```python
from build123d import *

# Parameters (mm, degrees)
SKETCH1_R             = 1.1
SKETCH1_R_2           = 3.75
BOSS_EXTRUDE1_DEPTH   = 2
F_1_0MM_DOWEL_HOLE1_D = 1
FILLET1_R             = 1


with BuildPart() as part:
    # Sketch1 → Boss-Extrude1 (new body)
    with BuildSketch(Plane.XY):
        with BuildLine():
            Line((-19.5, 2.7), (-6.306155873, 4.504985917))
            ThreePointArc((-6.306155873, 4.504985917), (0, 7.75), (6.306155873, 4.504985917))
            Line((6.306155873, 4.504985917), (19.5, 2.7))
            ThreePointArc((19.5, 2.7), (22.2, 0), (19.5, -2.7))
            Line((19.5, -2.7), (6.306155873, -4.504985917))
            ThreePointArc((6.306155873, -4.504985917), (0, -7.75), (-6.306155873, -4.504985917))
            Line((-6.306155873, -4.504985917), (-19.5, -2.7))
            ThreePointArc((-19.5, -2.7), (-22.2, 0), (-19.5, 2.7))
        make_face()
        with Locations((-19.5, 0)):
            Circle(SKETCH1_R, mode=Mode.SUBTRACT)
        with Locations(Location((19.5, 0, 0), (0, 0, 180))):
            Circle(SKETCH1_R, mode=Mode.SUBTRACT)
        Circle(SKETCH1_R_2, mode=Mode.SUBTRACT)
        with BuildLine():
            Line((-10, -0.75), (-15, -0.75))
            ThreePointArc((-15, -0.75), (-15.75, 0), (-15, 0.75))
            Line((-15, 0.75), (-10, 0.75))
            ThreePointArc((-10, 0.75), (-9.25, 0), (-10, -0.75))
        make_face(mode=Mode.SUBTRACT)
        with BuildLine():
            Line((10, -0.75), (15, -0.75))
            ThreePointArc((15, -0.75), (15.75, 0), (15, 0.75))
            Line((15, 0.75), (10, 0.75))
            ThreePointArc((10, 0.75), (9.25, 0), (10, -0.75))
        make_face(mode=Mode.SUBTRACT)
    extrude(amount=BOSS_EXTRUDE1_DEPTH)

    # Ø1.0mm Dowel Hole1 (through all)
    with Locations(Plane.XY.offset(2)):
        with Locations((-5.5, 0), (0, 5.5), (5.5, 0), (0, -5.5)):
            Hole(F_1_0MM_DOWEL_HOLE1_D / 2)

    # Fillet1
    fillet1_edges = [part.edges().sort_by_distance(p)[0] for p in [
        (-6.306155873, 4.504985917, 1),
        (6.306155873, 4.504985917, 1),
        (6.306155873, -4.504985917, 1),
        (-6.306155873, -4.504985917, 1),
    ]]
    fillet(fillet1_edges, radius=FILLET1_R)


solid = part.part
```
Geometry check sheet. Reference: the model listing, model coordinates, mm. A direction names the side the tool comes from. Coordinates: 2 decimals unless noted, no trailing zeros. Write each loop counter-clockwise with the first axis right and the second up, starting at its lowest first coordinate (ties: lowest second). Pieces come first, ordered by that corner, then holes. Notation, with made-up numbers: (67, 63) -> (76, 63) arc R25 cw to (76, 79) -> close; hole circle Ø6 at (-28.75, 31). An arc over 180 degrees is marked (long way). Use CSV: the item, a comma, the result in double quotes. Start each with the question number.
Item 1: Depth check by flat-ended pin: pin 1 Ø0.6 at (x, z) = (-11.5, 1) entering from -Y; pin 2 Ø1 at (x, z) = (13, 1) entering from -Y; pin 3 Ø3 at (x, y) = (-19.5, 0) entering from -Z; pin 4 Ø4.5 at (x, y) = (0, 0) entering from -Z. Enter the tip coordinate at first touch or a pass-through.
Item 2: Cross-section at B-B, the plane y = 0. State how many separate pieces and enclosed holes the cut face has, plus the area to 3 significant figures.
Item 3: Mould release check, pull along X, two halves, no side actions. Record for faces 1 (the flat face through (-13.02, -3.587, 0.986)), 2 (the cylindrical face through (-5, 0, 1)), 3 (the flat face through (-4.6, 0.1, 2)), 4 (the cylindrical face through (0.1, -7.75, 0.99)): released by +X, released by -X, zero draft, split by the parting line, or undercut.
Item 4: Cross-section at A-A, the plane x = 0. Record the cut outline in (y, z), plus the area to 3 significant figures.
Item 5: Set-up check for faces 5 (the cylindrical face through (-0.1, 7.75, 0.99)), 6 (the cylindrical face through (9.25, 0.02, 0.99)): record each of +Z, -Z, +X, -X, +Y, -Y from which the full face is reachable in a straight line by a thin tool's end or side.
Item 6: Thickness scan on line 1 (Y direction, x = 19.5, z = 0.2); line 2 (X direction, y = 2.25, z = 0.15); line 3 (Y direction, x = 19, z = 0.9). Record the ranges inside material, lowest first.
Item 7: Cross-section at D-D, the plane x = 12. Record the cut outline in (y, z), plus the area to 3 significant figures.
Answers:
1,pin 1,"y = -3.84"
1,pin 2,"y = -3.66"
1,pin 3,"z = 0"
1,pin 4,"through"
2,separate pieces,"8"
2,enclosed holes,"0"
2,area,"35.0 mm^2"
3,face 1,"released by -X"
3,face 2,"undercut"
3,face 3,"zero draft"
3,face 4,"split by the parting line"
4,outline,"(-7.75, 0) -> (-6, 0) -> (-6, 2) -> (-7.75, 2) -> close; (-5, 0) -> (-3.75, 0) -> (-3.75, 2) -> (-5, 2) -> close; (3.75, 0) -> (5, 0) -> (5, 2) -> (3.75, 2) -> close; (6, 0) -> (7.75, 0) -> (7.75, 2) -> (6, 2) -> close"
4,area,"12.0 mm^2"
5,face 5,"+Z, -Z, +Y"
5,face 6,"+Z, -Z"
6,line 1,"-2.7 to -1.1, 1.1 to 2.7"
6,line 2,"-20.99 to -3, 3 to 20.99"
6,line 3,"-2.77 to -0.98, 0.98 to 2.77"
7,outline,"(-3.73, 0) -> (-0.75, 0) -> (-0.75, 2) -> (-3.73, 2) -> close; (0.75, 0) -> (3.73, 0) -> (3.73, 2) -> (0.75, 2) -> close"
7,area,"11.9 mm^2"
